The listing builds one solid part. Answer for the finished solid, in the listing's coordinates (mm). Give positions to 0.01 mm unless a question says otherwise; leave off trailing zeros. Loops run counter-clockwise (first coordinate to the right, second up) from the corner with the lowest first, then second, coordinate; pieces in that order, holes last.
Item 1: Section B-B, the plane x = -54.5 is taken. Give the vertices of the cut face in (y, z), and give its area (3 significant figures).
Item 2: Section D-D, the plane y = -58 is taken. Give the vertices of the cut face in (x, z).
Item 3: The mould has two halves that part along Y. Classify faces 1 (the face through (-61, 0, 1)), 2 (the face through (-1, 1, 0)): pulls with the +Y half, pulls with the -Y half, needs draft (parallel to the pull), parting line crosses it, or undercut.
Item 4: Section C-C, the plane z = 2.3 is taken. Give the number of separate pieces and of enclosed holes in the cut face, and give its area (3 significant figures).
Item 5: Section A-A, the plane y = 0 is taken. Give the vertices of the cut face in (x, z), and give its area (3 significant figures).
Item 6: Consider line 1 along Y through (x, z) = (-12.5, 2); line 2 along X through (y, z) = (-17, 1.3); line 3 along Y through (x, z) = (-42, 1.65). Determine where each line is inside the solid, lowest interval first.
Item 7: Each of these flat-tipped pins is pushed along its axis until it touches: pin 1 Ø1.5 at (x, z) = (33.5, 1) entering from +Y; pin 2 Ø1.5 at (y, z) = (5.5, 2) entering from -X; pin 3 Ø1.5 at (y, z) = (4, 1.5) entering from +X. Where does it stop, or does it pass through?
from build123d import *

# Parameters (mm, degrees)
CROQUIS1_R              = 65
CROQUIS1_R_2            = 1.75
CROQUIS1_W              = 20
CROQUIS1_H              = 20
CROQUIS1_W_2            = 25
CROQUIS1_H_2            = 14
CROQUIS1_W_3            = 30
CROQUIS1_H_3            = 25
CROQUIS1_W_4            = 3
CROQUIS1_W_5            = 7
CROQUIS1_H_4            = 7
SALIENTE_EXTRUIR1_DEPTH = 3
CROQUIS2_R              = 1.75
CORTAR_EXTRUIR1_DEPTH   = 3


with BuildPart() as part:
    # Croquis1 → Saliente-Extruir1 (new body)
    with BuildSketch(Plane.XY):
        Circle(CROQUIS1_R)
        with Locations((-12.5, 17)):
            Circle(CROQUIS1_R_2, mode=Mode.SUBTRACT)
        with Locations((12.5, 17)):
            Circle(CROQUIS1_R_2, mode=Mode.SUBTRACT)
        with Locations(Location((12.5, -17, 0), (0, 0, 180))):
            Circle(CROQUIS1_R_2, mode=Mode.SUBTRACT)
        with Locations(Location((-12.5, -17, 0), (0, 0, 180))):
            Circle(CROQUIS1_R_2, mode=Mode.SUBTRACT)
        with Locations((-20, 0)):
            Rectangle(CROQUIS1_W, CROQUIS1_H, mode=Mode.SUBTRACT)
        with Locations((-48.5, 0)):
            Rectangle(CROQUIS1_W_2, CROQUIS1_H_2, mode=Mode.SUBTRACT)
        with Locations((25, 0)):
            Rectangle(CROQUIS1_W_3, CROQUIS1_H_3, mode=Mode.SUBTRACT)
        with Locations((46.5, 0)):
            Rectangle(CROQUIS1_W_4, CROQUIS1_H_2, mode=Mode.SUBTRACT)
        with Locations((55.5, 0)):
            Rectangle(CROQUIS1_W_5, CROQUIS1_H_4, mode=Mode.SUBTRACT)
    extrude(amount=SALIENTE_EXTRUIR1_DEPTH)

    # Croquis2 → Cortar-Extruir1 (cut)
    with BuildSketch(Plane.XY.offset(3)):
        with Locations((-42, 44)):
            Circle(CROQUIS2_R)
        with Locations((18, 58)):
            Circle(CROQUIS2_R)
        with Locations(Location((18, -58, 0), (0, 0, 180))):
            Circle(CROQUIS2_R)
        with Locations(Location((-42, -44, 0), (0, 0, 180))):
            Circle(CROQUIS2_R)
    extrude(amount=-CORTAR_EXTRUIR1_DEPTH, mode=Mode.SUBTRACT)


solid = part.part
Worked answers:
1. outline: (-35.42, 0) - (-7, 0) - (-7, 3) - (-35.42, 3) - close; (7, 0) - (35.42, 0) - (35.42, 3) - (7, 3) - close
1. area: 171 mm2
2. outline: (-29.34, 0) - (16.25, 0) - (16.25, 3) - (-29.34, 3) - close; (19.75, 0) - (29.34, 0) - (29.34, 3) - (19.75, 3) - close
3. face 1: undercut
3. face 2: needs draft
4. separate pieces: 1
4. enclosed holes: 13
4. area: 11,600 mm2
5. outline: (-65, 0) - (-61, 0) - (-61, 3) - (-65, 3) - close; (-36, 0) - (-30, 0) - (-30, 3) - (-36, 3) - close; (-10, 0) - (10, 0) - (10, 3) - (-10, 3) - close; (40, 0) - (45, 0) - (45, 3) - (40, 3) - close; (48, 0) - (52, 0) - (52, 3) - (48, 3) - close; (59, 0) - (65, 0) - (65, 3) - (59, 3) - close
5. area: 135 mm2
6. line 1: y = -63.79 to -18.75, -15.25 to -10, 10 to 15.25, 18.75 to 63.79
6. line 2: x = -62.74 to -14.25, -10.75 to 10.75, 14.25 to 62.74
6. line 3: y = -49.61 to -45.75, -42.25 to -7, 7 to 42.25, 45.75 to 49.61
7. pin 1: stops at y = 56.15
7. pin 2: stops at x = -64.83
7. pin 3: stops at x = 64.92
